Build history of the part. All positions in model axes, mm. A direction names the side the tool comes from. Round coordinates to 2 decimals unless told otherwise and drop trailing zeros. Order: outer loops, then holes, each group sorted by start corner. A loop starts at its lowest first (then second) coordinate and runs counter-clockwise, first axis right, second up. Notation, with made-up numbers: M -27.5,2.25 L 11.5,2.25 A20 ccw 11.5,18.25 Z; hole C 13,64.5 d7. An arc over 180 degrees is marked long. Use CSV: the item, a comma, the result in double quotes.
from build123d import *

# Parameters (mm, degrees)
F1_DEPTH = 10
F3_DEPTH = 0.5
F4_R     = 0.3
F5_W     = 1
F5_H     = 10
F6_DEPTH = 5.5
F7_R     = 0.4
F8_DEPTH = 12.001


# Not quite as in the source:
# - a feature names something its author has since deleted; it is built from what else it names


with BuildPart() as f1:
    # F0 (on Front) → F1 (new body)
    with BuildSketch(Plane.XZ):
        with BuildLine():
            Line((-6, 9), (-6, 0))
            Line((-6, 0), (-1.6, 0))
            Line((-1.6, 0), (-1.6, 4))
            ThreePointArc((-1.6, 4), (0, 5.6), (1.6, 4))
            Line((1.6, 4), (1.6, 0))
            Line((1.6, 0), (6, 0))
            Line((6, 0), (6, 9))
            Line((6, 9), (-6, 9))
        make_face()
    extrude(amount=F1_DEPTH)

    # F2 (on face) → F3 (join)
    with BuildSketch(Plane(origin=(1.6, 0, 0), x_dir=(0, -1, 0), z_dir=(-1, 0, 0))):
        Polygon((5.1838214056, 6), (3, 0), (3.7, 0), (5.8838214056, 6), align=None)
        Polygon((6, 0), (6.7, 0), (8.8838214056, 6), (8.1838214056, 6), align=None)
    extrude(amount=F3_DEPTH)

    # F4
    f4_edges = [f1.edges().sort_by_distance(p)[0] for p in [
        (1.1, -3.939388, 2.580948),
        (1.1, -4.639388, 2.580948),
        (1.1, -6.939388, 2.580948),
        (1.1, -7.639388, 2.580948),
    ]]
    fillet(f4_edges, radius=F4_R)

    # F5 (on face) → F6 (cut)
    with BuildSketch(Plane(origin=(0, 0, 0), x_dir=(1, 0, 0), z_dir=(0, 0, -1))):
        with Locations((3.1, 5)):
            Rectangle(F5_W, F5_H)
    extrude(amount=-F6_DEPTH, mode=Mode.SUBTRACT)

    # F7 (on face) → F8 (cut, through all)
    with BuildSketch(Plane(origin=(-6, 0, 0), x_dir=(0, -1, 0), z_dir=(-1, 0, 0))):
        with Locations((5, 7)):
            Circle(F7_R)
    extrude(amount=-F8_DEPTH, mode=Mode.SUBTRACT)


solid = f1.part
(1) Drop flat-ended pins along their axis: pin 1 (6 mm diameter, centred on x = 3, y = -6.5, fed in from -Z); pin 2 (0.5 mm diameter, centred on x = 3, y = -4.5, fed in from -Z). Give the stop position or say it passes through.
Answer block:
pin 1,"stops at z = 0"
pin 2,"stops at z = 5.5"
(2) Cut at D-D, the plane z = 3.25. Count the separate pieces of the cut face and the enclosed holes in it, and give its area (3 significant figures).
Answer block:
separate pieces,"3"
enclosed holes,"0"
area,"78.6 mm²"
(3) Tool access for faces 1 (the face through (1, 0, 6)), 2 (the face through (1.19, -4.025, 2.566)), 3 (the face through (-0.084, -4.948, 7.397)), 4 (the face through (3.6, -5, 3)), 5 (the face through (1.186, -4.534, 2.554)): list every direction of +Z, -Z, +X, -X, +Y, -Y with a clear straight run to the whole face (end or side of a thin tool).
Answer block:
face 1,"+Z, -Z, +X, -X, +Y"
face 2,"+Y"
face 3,"+X, -X"
face 4,"-Z, +Y, -Y"
face 5,"-Z"
(4) Cut at A-A, the plane z = 7. Give the cut face in (x, y), and give its area (3 significant figures).
Answer block:
outline,"M -6,-10 L 6,-10 L 6,-5.4 L -6,-5.4 Z; M -6,-4.6 L 6,-4.6 L 6,0 L -6,0 Z"
area,"110 mm²"
(5) Wall check: line 1 (X direction, y = -0.75, z = 1); line 2 (Z direction, x = -1.75, y = -5); line 3 (X direction, y = -7.25, z = 2.75). Give the ranges that are in metal, low to high. Write a range as from..to.
Answer block:
line 1,"x = -6..-1.6, 1.6..2.6, 3.6..6"
line 2,"z = 0..6.6, 7.4..9"
line 3,"x = -6..-1.6, 1.11..2.6, 3.6..6"
(6) Cut at C-C, the plane y = -9. Give the cut face in (x, z).
Answer block:
outline,"M -6,0 L -1.6,0 L -1.6,4 A1.6 cw 1.6,4 L 1.6,0 L 2.6,0 L 2.6,5.5 L 3.6,5.5 L 3.6,0 L 6,0 L 6,9 L -6,9 Z"
(7) Cut at B-B, the plane x = 0. Give the cut face in (y, z), and give its area (3 significant figures).
Answer block:
outline,"M -10,5.6 L 0,5.6 L 0,9 L -10,9 Z; hole C -5,7 d0.8"
area,"33.5 mm²"
(8) Two-plate mould, pull along Z, no slides. Class faces 6 (the face through (1.19, -7.025, 2.566)), 7 (the face through (1.6, -6, 2)), 8 (the face through (5, -5, 0)), 9 (the face through (1, -10, 6)): released by +Z, released by -Z, zero draft, split by the parting line, or undercut.
Answer block:
face 6,"undercut"
face 7,"undercut"
face 8,"released by -Z"
face 9,"zero draft"
